Input: part model. Units: mm. Frame: model coordinates. A direction names the side the tool comes from. Round coordinates to 2 decimals unless told otherwise and drop trailing zeros. Loops run counter-clockwise (first coordinate to the right, second up) from the corner with the lowest first, then second, coordinate; pieces in that order, holes last. Notation, with made-up numbers: (20.5, 4.25) -> (37.5, 4.25) arc R23 cw to (37.5, 18.25) -> close; hole circle Ø10 at (78.25, 59). An arc over 180 degrees is marked (long way). One line per question, with ' | ' between items. Start each with the question number.
Q1. Contact query for flat-ended pins moving along their axis: P1, Ø5, axis at x = 0, y = 0, coming from the -Z side; P2, Ø3, axis at x = 11, z = 48, coming from the +Y side; P3, Ø3, axis at x = 8, y = 4, coming from the -Z side; P4, Ø6, axis at y = -8, z = 73.5, coming from the +X side. Output: stop coordinate, or through.
Q2. Mould query, pull axis X, two halves, no side actions, for faces 5 (the face through (-7.7, -3.43, 89.7)), 6 (the face through (0, 0, 15)), 7 (the face through (0.88, 8.38, 89.7)). Classes: pulls with the +X half, pulls with the -X half, needs draft (parallel to the pull), parting line crosses it, or undercut.
Q3. Cut plane B-B on x = 13.25. Return loops of the section in (y, z), and give its area (3 significant figures).
Q4. Cut plane C-C on y = 10.75. Return loops of the section in (x, z).
Q5. Access query for faces 1 (the face through (1.032, 8.653, 84.437)), 2 (the face through (6.5, -6.5, 80)), 3 (the face through (-1.032, -8.653, 84.437)), 4 (the face through (6.98, -5.22, 84.44)). Directions: +Z, -Z, +X, -X, +Y, -Y. A direction counts if a zero-diameter tool reaches every point of the face in a straight line with its end or side. Return the directions, or none.
Q6. Material intervals for L1, parallel to Y at x = 0, z = 4.5; L2, parallel to Z at x = -12.5, y = 5.5; L3, parallel to Z at x = -1.5, y = -1.5, sorted ascending.
Q7. Cut plane A-A on z = 24. Return loops of the section in (x, y), and give its area (3 significant figures).
from build123d import *

# Parameters (mm, degrees)
SKETCH1_R           = 15
BOSS_EXTRUDE1_DEPTH = 80
SKETCH2_R           = 4
CUT_EXTRUDE1_DEPTH  = 15
BOSS_EXTRUDE2_DEPTH = 10
FILLET1_R           = 1


with BuildPart() as part:
    # Sketch1 → Boss-Extrude1 (new body)
    with BuildSketch(Plane.XY):
        Circle(SKETCH1_R)
    extrude(amount=BOSS_EXTRUDE1_DEPTH)

    # Sketch2 → Cut-Extrude1 (cut)
    with BuildSketch(Plane(origin=(0, 0, 0), x_dir=(-1, 0, 0), z_dir=(0, 0, -1))):
        Circle(SKETCH2_R)
    extrude(amount=-CUT_EXTRUDE1_DEPTH, mode=Mode.SUBTRACT)

    # Sketch4 → Boss-Extrude2 (add)
    with BuildSketch(Plane.XY.offset(80)):
        Polygon((5.969749807, 8.100368726), (-4.030250193, 9.22013935), (-10, 1.119770624), (-5.969749807, -8.100368726), (4.030250193, -9.22013935), (10, -1.119770624), align=None)
    extrude(amount=BOSS_EXTRUDE2_DEPTH)

    # Fillet1
    fillet1_edges = [part.edges().sort_by_distance(p)[0] for p in [
        (10, -1.119770624, 85),
        (5.969749807, 8.100368726, 85),
        (-4.030250193, 9.22013935, 85),
        (-10, 1.119770624, 85),
        (-5.969749807, -8.100368726, 85),
        (4.030250193, -9.22013935, 85),
        (7.984874903, 3.490299051, 90),
        (0.969749807, 8.660254038, 90),
        (-7.015125097, 5.169954987, 90),
        (-7.984874903, -3.490299051, 90),
        (-0.969749807, -8.660254038, 90),
        (7.015125097, -5.169954987, 90),
    ]]
    fillet(fillet1_edges, radius=FILLET1_R)


solid = part.part
Results:
1) P1: z = 15 | P2: y = 11.61 | P3: z = 0 | P4: x = 14.14
2) face 5: pulls with the -X half | face 6: undercut | face 7: pulls with the +X half
3) outline: (-7.03, 0) -> (7.03, 0) -> (7.03, 80) -> (-7.03, 80) -> close | area: 1,120 mm^2
4) outline: (-10.46, 0) -> (10.46, 0) -> (10.46, 80) -> (-10.46, 80) -> close
5) face 1: +Z, +X, +Y | face 2: +Z | face 3: +Z, -X, -Y | face 4: +Z, +X, -Y
6) L1: -15 to -4, 4 to 15 | L2: 0 to 80 | L3: 15 to 90
7) outline: circle Ø30 at (0, 0) | area: 707 mm^2
